from build123d import *

# Parameters (mm, degrees)
SKETCH_1_R      = 8.35
EXTRUDE_1_DEPTH = 17
FILLET_1_R      = 1
EXTRUDE_2_DEPTH = 0.3
SKETCH_3_W      = 3
SKETCH_3_H      = 0.3
EXTRUDE_3_DEPTH = 5


with BuildPart() as part:
    # Эскиз1 → Бобышка-Вытянуть1 (new, symmetric)
    with BuildSketch(Plane(origin=(0, 0, 0), x_dir=(0, 0, -1), z_dir=(1, 0, 0))):
        Circle(SKETCH_1_R)
    extrude(amount=EXTRUDE_1_DEPTH, both=True)

    # Скругление1
    fillet_1_edges = [part.edges().sort_by_distance(p)[0] for p in [
        (-17, 0, 8.35),
        (17, 0, 8.35),
    ]]
    fillet(fillet_1_edges, radius=FILLET_1_R)

    # Эскиз2 → Бобышка-Вытянуть2 (add)
    with BuildSketch(Plane(origin=(17, 0, 0), x_dir=(0, 0, -1), z_dir=(1, 0, 0))):
        with BuildLine():
            Line((-1.5, -9.35), (1.5, -9.35))
            Line((1.5, -9.35), (1.5, -7.195310973))
            ThreePointArc((1.5, -7.195310973), (0, -7.35), (-1.5, -7.195310973))
            Line((-1.5, -7.195310973), (-1.5, -9.35))
        make_face()
    extrude_2 = extrude(amount=-EXTRUDE_2_DEPTH)

    # Эскиз3 → Бобышка-Вытянуть3 (add)
    with BuildSketch(Plane(origin=(17, 0, 0), x_dir=(0, 0, -1), z_dir=(1, 0, 0))):
        with Locations((0, -9.2)):
            Rectangle(SKETCH_3_W, SKETCH_3_H)
    extrude_3 = extrude(amount=EXTRUDE_3_DEPTH)

    # Зеркальное отражение1: Бобышка-Вытянуть2, Бобышка-Вытянуть3 across plane
    add(extrude_2.mirror(Plane(origin=(0, 0, 0), x_dir=(0, 0, 1), z_dir=(1, 0, 0))))
    add(extrude_3.mirror(Plane(origin=(0, 0, 0), x_dir=(0, 0, 1), z_dir=(1, 0, 0))))


solid = part.part
Model file for the job. Use its own axes, mm. A direction names the side the tool comes from. Give positions to 0.01 mm unless a question says otherwise; leave off trailing zeros. Order: outer loops, then holes, each group sorted by start corner. A loop starts at its lowest first (then second) coordinate and runs counter-clockwise, first axis right, second up. Notation, with made-up numbers: M 21,-7.5 L 73,-7.5 A32 cw 73,27.5 Z; hole C 38,74 d6. An arc over 180 degrees is marked long. Put each result on its own line as item: value. Start each with the question number.
(1) Pull direction X, two halves, no side cores. Call faces 1 (the face through (16.7, -9, 0)), 2 (the face through (17, -1, 0)), 3 (the face through (19, -9.05, 0)), 4 (the face through (-17, -1, 0)): released by +X, released by -X, zero draft, split by the parting line, or undercut.
(2) Band-saw the part on A-A on y = 0. Give the cut face in (x, z).
(3) Band-saw the part on B-B on z = 0. Give the cut face in (x, y), then the cut area to 3 significant figures.
(4) Tool access for faces 5 (the face through (-19, -9.35, 0)), 6 (the face through (-19, -9.05, 0)): list every direction of +Z, -Z, +X, -X, +Y, -Y with a clear straight run to the whole face (end or side of a thin tool).
(5) Drill centre lines: L1, parallel to X at y = 2.5, z = -5.25; L2, parallel to X at y = 4, z = 7; L3, parallel to Z at x = -6, y = 6.5. Where is each one in solid material? Low to high. Write a range as [from, to].
(6) Band-saw the part on C-C on x = -14.5. Give the cut face in (y, z).
(7) Pin check, flat tips, straight feed: pin 1 Ø0.7 at (y, z) = (-8.5, 0.5) entering from -X; pin 2 Ø2 at (x, y) = (-15.5, -3.5) entering from -Z; pin 3 Ø3 at (x, z) = (11.5, 5.5) entering from -Y; pin 4 Ø8 at (x, y) = (4, 3.5) entering from +Z. Stop position of each tip, or through.
Results below:
1. face 1: undercut
1. face 2: released by +X
1. face 3: zero draft
1. face 4: released by -X
2. outline: M -17,-7.35 A1 ccw -16,-8.35 L 16,-8.35 A1 ccw 17,-7.35 L 17,7.35 A1 ccw 16,8.35 L -16,8.35 A1 ccw -17,7.35 Z
3. outline: M -22,-9.35 L -16.7,-9.35 L -16.7,-8.06 A1 ccw -16,-8.35 L 16,-8.35 A1 ccw 16.7,-8.06 L 16.7,-9.35 L 22,-9.35 L 22,-9.05 L 17,-9.05 L 17,7.35 A1 ccw 16,8.35 L -16,8.35 A1 ccw -17,7.35 L -17,-9.05 L -22,-9.05 Z
3. area: 571 mm2
4. face 5: +Z, -Z, +X, -X, -Y
4. face 6: +Z, -Z, -X, +Y
5. L1: x = [-17, 17]
5. L2: x = [-16.7, 16.7]
5. L3: z = [-5.24, 5.24]
6. outline: C 0,0 d16.7
7. pin 1: stops at x = -17
7. pin 2: stops at z = -7.97
7. pin 3: stops at y = -7.33
7. pin 4: stops at z = 8.35
